from build123d import *

# Parameters (mm, degrees)
F0_W     = 609.6
F0_H     = 914.4
F0_R     = 9.525
F1_DEPTH = 152.4
F2_R     = 50.8
F3_R     = 25.4


with BuildPart() as f1:
    # F0 (on Front) → F1 (new body)
    with BuildSketch(Plane.XZ):
        with Locations((-104.6087741801, -270.9774990136)):
            Rectangle(F0_W, F0_H)
        with Locations((-358.6087741801, -639.2774990136)):
            Circle(F0_R, mode=Mode.SUBTRACT)
        with Locations((149.3912258199, -639.2774990136)):
            Circle(F0_R, mode=Mode.SUBTRACT)
        with Locations((-358.6087741801, 97.3225009864)):
            Circle(F0_R, mode=Mode.SUBTRACT)
        with Locations((149.3912258199, 97.3225009864)):
            Circle(F0_R, mode=Mode.SUBTRACT)
    extrude(amount=F1_DEPTH)

    # F2
    f2_edges = [f1.edges().sort_by_distance(p)[0] for p in [
        (200.191226, -76.2, -728.177499),
        (200.191226, -76.2, 186.222501),
        (-409.408774, -76.2, -728.177499),
        (-409.408774, -76.2, 186.222501),
    ]]
    fillet(f2_edges, radius=F2_R)

    # F3
    f3_edges = [f1.edges().sort_by_distance(p)[0] for p in [
        (-409.408774, -152.4, -270.977499),
        (-394.529799, -152.4, -713.298523),
        (-104.608774, -152.4, -728.177499),
        (185.31225, -152.4, -713.298523),
        (200.191226, -152.4, -270.977499),
        (-104.608774, -152.4, 186.222501),
        (185.31225, -152.4, 171.343525),
        (-394.529799, -152.4, 171.343525),
    ]]
    fillet(f3_edges, radius=F3_R)


solid = f1.part
The listing builds one solid part. Answer for the finished solid, in the listing's coordinates (mm). Give positions to 0.01 mm unless a question says otherwise; leave off trailing zeros. Use one line per item in the form item = value.
1) Consider probe 1 along Z at (x, y) = (-277, -141); probe 2 along X at (y, z) = (-144.5, -308); probe 3 along Z at (x, y) = (-179.5, -140). Determine where each line is inside the solid, lowest interval first. Write a range as [from, to].
Verdict:
probe_1 = [-723.97, 182.02]
probe_2 = [-402.42, 193.2]
probe_3 = [-724.6, 182.64]
2) Each of these flat-tipped pins is pushed along its axis until it touches: pin 1 (3 mm diameter, centred on x = 11.5, y = -135, fed in from -Z); pin 2 (2 mm diameter, centred on x = -254, y = -132, fed in from +Z); pin 3 (1 mm diameter, centred on x = 126.5, z = -106, fed in from +Y). Where does it stop, or does it pass through?
Verdict:
pin_1 = -727.33
pin_2 = 185.91
pin_3 = 0
3) The mould has two halves that part along Z. Classify faces 1 (the cylindrical face through (184.915, -64.389, -713.691)), 2 (the cylindrical face through (-101.05, -144.76, 178.98)), 3 (the cylindrical face through (139.875, -75.133, 97.741)): released by +Z, released by -Z, zero draft, split by the parting line, or undercut.
Verdict:
face_1 = released by -Z
face_2 = released by +Z
face_3 = undercut
